Read the model definition and answer for the solid it produces. Units are mm, in the model's axes. A direction names the side the tool comes from. Give positions to 0.01 mm unless a question says otherwise; leave off trailing zeros. Order: outer loops, then holes, each group sorted by start corner. A loop starts at its lowest first (then second) coordinate and runs counter-clockwise, first axis right, second up. Notation, with made-up numbers: (58.5, 86) -> (113.5, 86) arc R13 cw to (113.5, 106) -> close; hole circle Ø11 at (42.5, 41). An arc over 180 degrees is marked (long way). Use one line per item in the form item = value.
```python
from build123d import *

# Parameters (mm, degrees)
IZIM1_R                     = 2.5
Y_KSEKLIK_EKSTR_ZYON1_DEPTH = 10
RADYUS1_R                   = 7.5
RADYUS2_R                   = 7.5
KES_EKSTR_ZYON1_DEPTH       = 10
KES_EKSTR_ZYON2_DEPTH       = 2


with BuildPart() as part:
    # Çizim1 → Yükseklik-Ekstrüzyon1 (new body)
    with BuildSketch(Plane.XY):
        Polygon((-26.066455833, 76.796612605), (-11.294339538, 74.19188994), (28.705660462, 4.909857637), (28.705660462, -25.090142363), (3.705660462, -68.391412552), (-20.914533363, -64.05020811), (-8.101071955, -25.090142363), (-28.390881377, -25.090142363), (-28.390881377, 4.909857637), (-13.390881377, 4.909857637), align=None)
        with Locations((-23.390881377, -2.590142363)):
            Circle(IZIM1_R, mode=Mode.SUBTRACT)
        with Locations((-23.390881377, -17.590142363)):
            Circle(IZIM1_R, mode=Mode.SUBTRACT)
    extrude(amount=Y_KSEKLIK_EKSTR_ZYON1_DEPTH)

    # Radyus1
    radyus1_edges = [part.edges().sort_by_distance(p)[0] for p in [
        (-11.294339538, 74.19188994, 5),
    ]]
    fillet(radyus1_edges, radius=RADYUS1_R)

    # Radyus2
    radyus2_edges = [part.edges().sort_by_distance(p)[0] for p in [
        (28.705660462, 4.909857637, 5),
        (28.705660462, -25.090142363, 5),
        (3.705660462, -68.391412552, 5),
    ]]
    fillet(radyus2_edges, radius=RADYUS2_R)

    # Çizim2 → Kes-Ekstrüzyon1 (cut)
    with BuildSketch(Plane.XY.offset(10)):
        with BuildLine():
            Line((-15.434488962, 59.690510809), (-8.698721777, 21.490076831))
            ThreePointArc((-8.698721777, 21.490076831), (-7.843671419, 20.009086168), (-6.236702395, 19.424197275))
            Line((-6.236702395, 19.424197275), (7.335421508, 19.424197275))
            ThreePointArc((7.335421508, 19.424197275), (9.500485018, 20.674197275), (9.500485018, 23.174197275))
            Line((9.500485018, 23.174197275), (-10.56271444, 57.924678099))
            ThreePointArc((-10.56271444, 57.924678099), (-11.293836859, 58.72255821), (-12.293657506, 59.136697482))
            Line((-12.293657506, 59.136697482), (-15.434488962, 59.690510809))
        make_face()
        with BuildLine():
            Line((-8.242164507, -58.66898906), (-1.887676329, -59.789456774))
            ThreePointArc((-1.887676329, -59.789456774), (-0.39701023, -59.593206859), (0.711507625, -58.577437392))
            Line((0.711507625, -58.577437392), (13.550215896, -36.340142363))
            ThreePointArc((13.550215896, -36.340142363), (13.550215896, -33.840142363), (11.385152387, -32.590142363))
            Line((11.385152387, -32.590142363), (-0.86299285, -32.590142363))
            ThreePointArc((-0.86299285, -32.590142363), (-2.328828905, -33.064969615), (-3.237849836, -34.309082635))
            Line((-3.237849836, -34.309082635), (-10.182901048, -55.42590995))
            ThreePointArc((-10.182901048, -55.42590995), (-9.953266447, -57.490722349), (-8.242164507, -58.66898906))
        make_face()
    extrude(amount=-KES_EKSTR_ZYON1_DEPTH, mode=Mode.SUBTRACT)

    # Çizim3 → Kes-Ekstrüzyon2 (cut)
    with BuildSketch(Plane.XY.offset(10)):
        Polygon((-17, 71.667807617), (-15, 71.667807617), (-15, 69.167807617), (-12.5, 69.167807617), (-12.5, 67.167807617), (-15, 67.167807617), (-15, 64.667807617), (-17, 64.667807617), (-17, 67.167807617), (-19.5, 67.167807617), (-19.5, 69.167807617), (-17, 69.167807617), align=None)
    extrude(amount=-KES_EKSTR_ZYON2_DEPTH, mode=Mode.SUBTRACT)


solid = part.part
```
Item 1: Which of the six approach directions +Z, -Z, +X, -X, +Y, -Y give full straight-line access (tool end or side, diameter ignored) to faces 4 (the flat face through (-11.05, -65.79, 4.93)), 5 (the cylindrical face through (-2.31, -33.05, 5.07))?
Checks:
face_4 = +Z, -Z, -X, -Y
face_5 = +Z, -Z
Item 2: The part is cut by section B-B on y = 34. Give the vertices of the cut face in (x, z), and give its area (3 significant figures).
Checks:
outline = (-18.52, 0) -> (-10.9, 0) -> (-10.9, 10) -> (-18.52, 10) -> close; (3.25, 0) -> (11.91, 0) -> (11.91, 10) -> (3.25, 10) -> close
area = 163 mm²
Item 3: Straight lines are drawn through the part: L1, parallel to Y at x = 2.5, z = 5.75; L2, parallel to Y at x = 0.5, z = 6; L3, parallel to X at y = 3.5, z = 6.5. For each, find the intervals that lie inside material, in ascending order. Write a range as from..to.
Checks:
L1 = -67.1..-55.48, -32.59..19.42, 35.3..50.3
L2 = -67.56..-58.89, -32.59..19.42, 38.76..53.76
L3 = -28.39..28.68
Item 4: Determine the mould class of faces 1 (the cylindrical face through (28.443, 4.868, 5.07)), 2 (the flat face through (-18, -25.09, 5)), 3 (the cylindrical face through (-7.862, 20.025, 5.07)) for opening direction X: +X half, -X half, draft (parallel to the pull), parting line (faces both ways), or undercut.
Checks:
face_1 = +X half
face_2 = draft
face_3 = undercut
Item 5: The part is cut by section D-D on y = -40.5. Give the vertices of the cut face in (x, z).
Checks:
outline = (-13.17, 0) -> (-5.27, 0) -> (-5.27, 10) -> (-13.17, 10) -> close; (11.15, 0) -> (19.81, 0) -> (19.81, 10) -> (11.15, 10) -> close
Item 6: Given pin 1 Ø5 at (x, z) = (1, 5.5) entering from +Y; pin 2 Ø5 at (x, z) = (8, 5.5) entering from -Y; pin 3 Ø2 at (x, z) = (-18, 8.5) entering from +Y, each flat-ended and moving along its own axis, determine where each tip first touches the part or whether it passes through.
Checks:
pin_1 = 57.23
pin_2 = -65.01
pin_3 = 75.55
Item 7: The part is cut by section C-C on z = 3.25. State how many separate pieces and enclosed holes the cut face has, and give its area (3 significant figures).
Checks:
separate_pieces = 1
enclosed_holes = 4
area = 4,080 mm²
Item 8: The part is cut by section A-A on x = 2.5. Give the vertices of the cut face in (y, z), and give its area (3 significant figures).
Checks:
outline = (-67.1, 0) -> (-55.48, 0) -> (-55.48, 10) -> (-67.1, 10) -> close; (-32.59, 0) -> (19.42, 0) -> (19.42, 10) -> (-32.59, 10) -> close; (35.3, 0) -> (50.3, 0) -> (50.3, 10) -> (35.3, 10) -> close
area = 786 mm²
